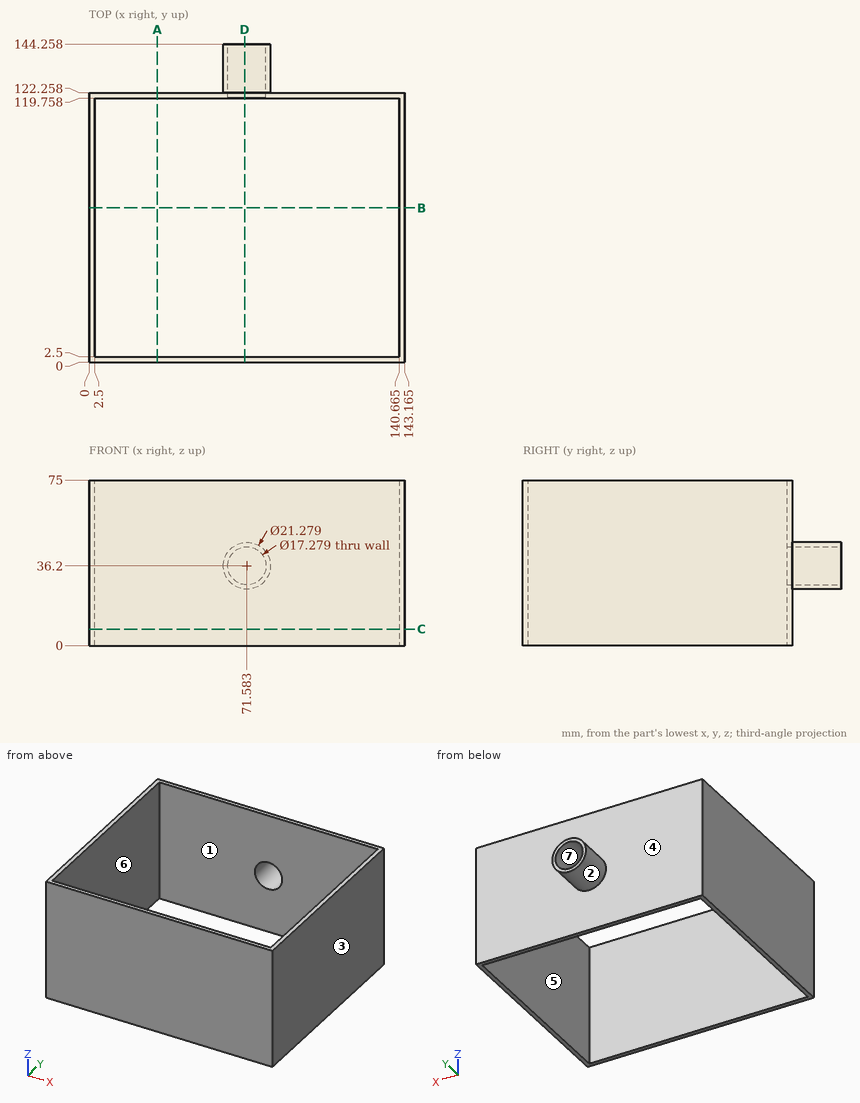
Design review of the part shown in the three views and the two pictorial views. Dimensions are in mm from the part's minimum x, y and z. A direction names the side the tool comes from. Give positions to 0.01 mm unless a question says otherwise; leave off trailing zeros. Write each loop counter-clockwise with the first axis right and the second up, starting at its lowest first coordinate (ties: lowest second). Pieces come first, ordered by that corner, then holes.
(1) Clearance check with a flat-ended pin moving along its axis: pin 1 Ø2 at (x, z) = (93, 38) entering from +Y. State where the tip first meets the part, or that it passes through.
Checked values:
pin 1: stops at y = 122.26
(2) Add section A-A (x = 31). Give the boundary of the cut face in (y, z), and give its area (3 significant figures).
Checked values:
outline: (0, 0) - (2.5, 0) - (2.5, 75) - (0, 75) - close; (119.76, 0) - (122.26, 0) - (122.26, 75) - (119.76, 75) - close
area: 375 mm2
(3) Mouldability with a two-part tool opening along Y and no side actions: class the marked faces 4, 5, 6 and 7 as +Y half, -Y half, draft (parallel to the pull), parting line (faces both ways), or undercut.
Checked values:
face 4: +Y half
face 5: undercut
face 6: undercut
face 7: draft
(4) Add section B-B (y = 70). Give the boundary of the cut face in (x, z) (1 decimal), and give its area (3 significant figures).
Checked values:
outline: (0, 0) - (2.5, 0) - (2.5, 75) - (0, 75) - close; (140.7, 0) - (143.2, 0) - (143.2, 75) - (140.7, 75) - close
area: 375 mm2
(5) Add section D-D (x = 70.5). Give the boundary of the cut face in (y, z) (1 decimal).
Checked values:
outline: (0, 0) - (2.5, 0) - (2.5, 75) - (0, 75) - close; (119.8, 0) - (122.3, 0) - (122.3, 25.6) - (144.3, 25.6) - (144.3, 27.6) - (119.8, 27.6) - close; (119.8, 44.8) - (144.3, 44.8) - (144.3, 46.8) - (122.3, 46.8) - (122.3, 75) - (119.8, 75) - close
(6) Wall thickness on line 1 along X through (y, z) = (69.5, 65.5) (1 decimal); line 2 along Y through (x, z) = (7, 62.5); line 3 along X through (y, z) = (130, 31) (1 decimal): over which ranges is each line inside the solid? List them lowest first.
Checked values:
line 1: x = 0 to 2.5, 140.7 to 143.2
line 2: y = 0 to 2.5, 119.76 to 122.26
line 3: x = 62.3 to 64.7, 78.5 to 80.9
(7) Add section C-C (z = 7.5). Give the boundary of the cut face in (x, y) (1 decimal), and give its area (3 significant figures).
Checked values:
outline: (0, 0) - (143.2, 0) - (143.2, 122.3) - (0, 122.3) - close; hole (2.5, 2.5) - (140.7, 2.5) - (140.7, 119.8) - (2.5, 119.8) - close
area: 1,300 mm2
(8) Tool access review of the marked faces 1, 2 and 3: name each direction out of +Z, -Z, +X, -X, +Y, -Y from which nothing blocks a thin tool from reaching the whole face with its end or side.
Checked values:
face 1: +Z, -Z
face 2: +Y
face 3: +Z, -Z, +X, +Y, -Y
